Part model, mm, in its own coordinate system. A direction names the side the tool comes from. Round coordinates to 2 decimals unless told otherwise and drop trailing zeros. Loops run counter-clockwise (first coordinate to the right, second up) from the corner with the lowest first, then second, coordinate; pieces in that order, holes last. Notation, with made-up numbers: (-30.5, 22.5) - (26.5, 22.5) arc R27 ccw to (26.5, 43.5) - close; hole circle Ø7 at (10, 56.5). An arc over 180 degrees is marked (long way). Put each result on its own line as item: value.
from build123d import *

# Parameters (mm, degrees)
SKETCH1_W                    = 69.85
SKETCH1_H                    = 44.45
SKETCH1_R                    = 4.1671875
BOSS_EXTRUDE1_DEPTH          = 23.749
CUT_EXTRUDE1_DEPTH           = 17.399
SKETCH3_OUTSIDE_W            = 89.076
SKETCH3_OUTSIDE_H            = 63.676
CUT_EXTRUDE2_DEPTH           = 23.749
SKETCH4_OUTSIDE_W            = 89.076
SKETCH4_OUTSIDE_H            = 63.676
CUT_EXTRUDE3_DEPTH           = 6.35
CUT_EXTRUDE4_DEPTH           = 87.132688342
SKETCH6_R                    = 7.1374
CUT_EXTRUDE6_DEPTH           = 6.35
CUT_EXTRUDE6_DRAFT           = -30
CUT_EXTRUDE6_PROFILE_2_DEPTH = 6.35
CUT_EXTRUDE6_PROFILE_2_DRAFT = -30
SKETCH7_W                    = 7.874
SKETCH7_H                    = 9.578750354
CUT_EXTRUDE7_DEPTH           = 85.602306121
FILLET2_R                    = 3.683
CHAMFER1_SIZE                = 0.508
FILLET3_R                    = 6.35
FILLET4_R                    = 3.175


with BuildPart() as part:
    # Sketch1 → Boss-Extrude1 (new body)
    with BuildSketch(Plane.XY):
        with Locations((-34.925, 22.225)):
            Rectangle(SKETCH1_W, SKETCH1_H)
        with Locations((-58.7375, 34.925)):
            Circle(SKETCH1_R, mode=Mode.SUBTRACT)
        with Locations((-11.1125, 34.925)):
            Circle(SKETCH1_R, mode=Mode.SUBTRACT)
    extrude(amount=-BOSS_EXTRUDE1_DEPTH)

    # Sketch2 → Cut-Extrude1 (cut)
    with BuildSketch(Plane.XY):
        with BuildLine():
            Line((-69.85, 36.957634205), (-69.85, 0))
            Line((-69.85, 0), (-34.925, 0))
            Line((-34.925, 0), (0, 0))
            Line((0, 0), (0, 36.957634205))
            ThreePointArc((0, 36.957634205), (-3.683397045, 29.404464031), (-11.902903765, 27.655892395))
            ThreePointArc((-11.902903765, 27.655892395), (-34.925, 30.48), (-57.947096235, 27.655892395))
            ThreePointArc((-57.947096235, 27.655892395), (-66.166602955, 29.404464031), (-69.85, 36.957634205))
        make_face()
    extrude(amount=-CUT_EXTRUDE1_DEPTH, mode=Mode.SUBTRACT)

    # Sketch3 outside → Cut-Extrude2 (cut)
    with BuildSketch(Plane.XY):
        with Locations((-34.925, 22.225)):
            Rectangle(SKETCH3_OUTSIDE_W, SKETCH3_OUTSIDE_H)
        with BuildLine():
            Line((-69.85, 36.83), (-69.85, 0))
            Line((-69.85, 0), (0, 0))
            Line((0, 0), (0, 36.83))
            ThreePointArc((0, 36.83), (-2.231846327, 42.218153673), (-7.62, 44.45))
            Line((-7.62, 44.45), (-62.23, 44.45))
            ThreePointArc((-62.23, 44.45), (-67.618153673, 42.218153673), (-69.85, 36.83))
        make_face(mode=Mode.SUBTRACT)
    extrude(amount=-CUT_EXTRUDE2_DEPTH, mode=Mode.SUBTRACT)

    # Sketch4 outside → Cut-Extrude3 (cut)
    with BuildSketch(Plane.XY.offset(-17.399)):
        with Locations((-34.925, 22.225)):
            Rectangle(SKETCH4_OUTSIDE_W, SKETCH4_OUTSIDE_H)
        with BuildLine():
            Line((-69.85, 44.45), (0, 44.45))
            Line((0, 44.45), (0, 15.875))
            ThreePointArc((0, 15.875), (-1.757438621, 9.877460267), (-6.473877678, 5.776938839))
            Line((-6.473877678, 5.776938839), (-19.05, 0))
            Line((-19.05, 0), (-50.8, 0))
            Line((-50.8, 0), (-63.376122322, 5.776938839))
            ThreePointArc((-63.376122322, 5.776938839), (-68.092561379, 9.877460267), (-69.85, 15.875))
            Line((-69.85, 15.875), (-69.85, 44.45))
        make_face(mode=Mode.SUBTRACT)
    extrude(amount=-CUT_EXTRUDE3_DEPTH, mode=Mode.SUBTRACT)

    # Sketch5 → Cut-Extrude4 (cut, through all)
    with BuildSketch(Plane.XY):
        with BuildLine():
            Line((-38.862, 34.22084733), (-38.862, 40.513))
            ThreePointArc((-38.862, 40.513), (-37.708879398, 43.296879398), (-34.925, 44.45))
            Line((-34.925, 44.45), (-50.673, 44.45))
            ThreePointArc((-50.673, 44.45), (-47.889120602, 43.296879398), (-46.736, 40.513))
            Line((-46.736, 40.513), (-46.736, 34.22084733))
            ThreePointArc((-46.736, 34.22084733), (-42.799, 30.28384733), (-38.862, 34.22084733))
        make_face()
        with BuildLine():
            Line((-19.177, 44.45), (-34.925, 44.45))
            ThreePointArc((-34.925, 44.45), (-32.141120602, 43.296879398), (-30.988, 40.513))
            Line((-30.988, 40.513), (-30.988, 34.22084733))
            ThreePointArc((-30.988, 34.22084733), (-27.051, 30.28384733), (-23.114, 34.22084733))
            Line((-23.114, 34.22084733), (-23.114, 40.513))
            ThreePointArc((-23.114, 40.513), (-21.960879398, 43.296879398), (-19.177, 44.45))
        make_face()
    extrude(amount=-CUT_EXTRUDE4_DEPTH, mode=Mode.SUBTRACT)


with BuildPart() as cut_extrude6_tool:
    # Sketch6 → Cut-Extrude6 (with draft: the straight prism first)
    with BuildSketch(Plane(origin=(0, 0, -23.749), x_dir=(-1, 0, 0), z_dir=(0, 0, -1))):
        with Locations((11.1125, 15.875)):
            Circle(SKETCH6_R)
    extrude(amount=-CUT_EXTRUDE6_DEPTH)
    # Cut-Extrude6: the draft: its side faces are tilted about the plane it starts from
    cut_extrude6_sides = [cut_extrude6_tool.faces().sort_by_distance(p)[0] for p in [
        (-3.9751, 15.875, -20.574),
    ]]
    draft(cut_extrude6_sides, Plane(origin=(0, 0, -23.749), x_dir=(-1, 0, 0), z_dir=(0, 0, -1)), CUT_EXTRUDE6_DRAFT)


with BuildPart() as part_1:
    add(part.part)

    # Cut-Extrude6: cut by cut_extrude6_tool
    add(cut_extrude6_tool.part, mode=Mode.SUBTRACT)


with BuildPart() as cut_extrude6_profile_2_tool:
    # Sketch6 → Cut-Extrude6 profile 2 (with draft: the straight prism first)
    with BuildSketch(Plane(origin=(0, 0, -23.749), x_dir=(-1, 0, 0), z_dir=(0, 0, -1))):
        with Locations((58.7375, 15.875)):
            Circle(SKETCH6_R)
    extrude(amount=-CUT_EXTRUDE6_PROFILE_2_DEPTH)
    # Cut-Extrude6 profile 2: the draft: its side faces are tilted about the plane it starts from
    cut_extrude6_profile_2_sides = [cut_extrude6_profile_2_tool.faces().sort_by_distance(p)[0] for p in [
        (-51.6001, 15.875, -20.574),
    ]]
    draft(cut_extrude6_profile_2_sides, Plane(origin=(0, 0, -23.749), x_dir=(-1, 0, 0), z_dir=(0, 0, -1)), CUT_EXTRUDE6_PROFILE_2_DRAFT)


with BuildPart() as part_2:
    add(part_1.part)

    # Cut-Extrude6 profile 2: cut by cut_extrude6_profile_2_tool
    add(cut_extrude6_profile_2_tool.part, mode=Mode.SUBTRACT)

    # Sketch7 → Cut-Extrude7 (cut, through all)
    with BuildSketch(Plane.XY.offset(-17.399)):
        with Locations((-42.799, 32.577548488)):
            Rectangle(SKETCH7_W, SKETCH7_H)
        with Locations((-27.051, 32.577548488)):
            Rectangle(SKETCH7_W, SKETCH7_H)
    extrude(amount=CUT_EXTRUDE7_DEPTH, mode=Mode.SUBTRACT)

    # Fillet2
    fillet2_edges = [part_2.edges().sort_by_distance(p)[0] for p in [
        (-38.862, 30.398600552, -8.6995),
        (-46.736, 29.744881257, -8.6995),
        (-23.114, 29.744881257, -8.6995),
        (-30.988, 30.398600552, -8.6995),
    ]]
    fillet(fillet2_edges, radius=FILLET2_R)

    # Chamfer1
    chamfer1_edges = [part_2.edges().sort_by_distance(p)[0] for p in [
        (-62.9046875, 34.925, -23.749),
        (-62.9046875, 34.925, 0),
        (-15.2796875, 34.925, -23.749),
        (-15.2796875, 34.925, 0),
    ]]
    chamfer(chamfer1_edges, length=CHAMFER1_SIZE)

    # Fillet3
    fillet3_edges = [part_2.edges().sort_by_distance(p)[0] for p in [
        (-50.8, 0, -20.574),
        (-19.05, 0, -20.574),
    ]]
    fillet(fillet3_edges, radius=FILLET3_R)

    # Fillet4
    fillet4_edges = [part_2.edges().sort_by_distance(p)[0] for p in [
        (-1.757438621, 9.877460267, -23.749),
        (-68.092561379, 9.877460267, -23.749),
        (-12.130971605, 3.178309088, -23.749),
        (-56.4515, 44.45, -23.749),
        (-42.799, 30.28384733, -23.749),
        (-47.889120602, 43.296879398, -23.749),
        (-34.925, 44.45, -23.749),
        (-38.862, 37.366923665, -23.749),
        (-46.736, 37.366923665, -23.749),
        (-23.114, 37.366923665, -23.749),
        (-27.051, 30.28384733, -23.749),
        (-21.960879398, 43.296879398, -23.749),
        (-30.988, 37.366923665, -23.749),
        (-57.719028395, 3.178309088, -23.749),
        (-34.925, 0, -23.749),
        (-19.082063244, 0.146612369, -23.749),
        (-50.767936756, 0.146612369, -23.749),
        (-69.85, 26.3525, -23.749),
        (-13.3985, 44.45, -23.749),
        (-2.231846327, 42.218153673, -23.749),
        (-67.618153673, 42.218153673, -23.749),
        (0, 26.3525, -23.749),
    ]]
    fillet(fillet4_edges, radius=FILLET4_R)


solid = part_2.part
1. Tool access for faces 1 (the cylindrical face through (-32.099, 31.527, -8.578)), 2 (the cylindrical face through (-31.9, 37.3, -22.8)), 3 (the cylindrical face through (-21.99, 43.27, -10.14)), 4 (the cylindrical face through (-67.559, 42.277, -10.143)): list every direction of +Z, -Z, +X, -X, +Y, -Y with a clear straight run to the whole face (end or side of a thin tool).
A:
face 1: +Z, -Y
face 2: -Z, +Y
face 3: +Z, -Z, +Y
face 4: +Z, -Z, -X, +Y
2. Probe line 1 along Y through (x, z) = (-11, -18.5); line 2 along Y through (x, z) = (-12, -17.75); line 3 along X through (y, z) = (39.5, -2.5). List the from-to ranges inside material, lowest first. Write a range as [from, to].
A:
line 1: y = [3.7, 11.77], [19.98, 30.76], [39.09, 44.45]
line 2: y = [3.24, 12.31], [19.44, 30.85], [39, 44.45]
line 3: x = [-69.37, -46.74], [-38.86, -30.99], [-23.11, -0.48]
3. Band-saw the part on B-B (y = 24). List the corners of the cut face in (x, z) (3 decimals), plus the area to 3 significant figures.
A:
outline: (-69.85, -20.574) arc R3.175 ccw to (-66.675, -23.749) - (-3.175, -23.749) arc R3.175 ccw to (0, -20.574) - (0, -17.399) - (-69.85, -17.399) - close
area: 439 mm²
4. Pin check, flat tips, straight feed: P1, Ø18.5, axis at x = -23, y = 22, coming from the +Z side; P2, Ø12, axis at y = 29, z = -4.5, coming from the -X side. Stop position of each tip, or through.
A:
P1: stops at z = 0
P2: stops at x = -69.65
5. Band-saw the part on A-A (z = -11.5). Give the number of separate pieces and of enclosed holes in the cut face, plus the area to 3 significant figures.
A:
separate pieces: 3
enclosed holes: 2
area: 670 mm²
